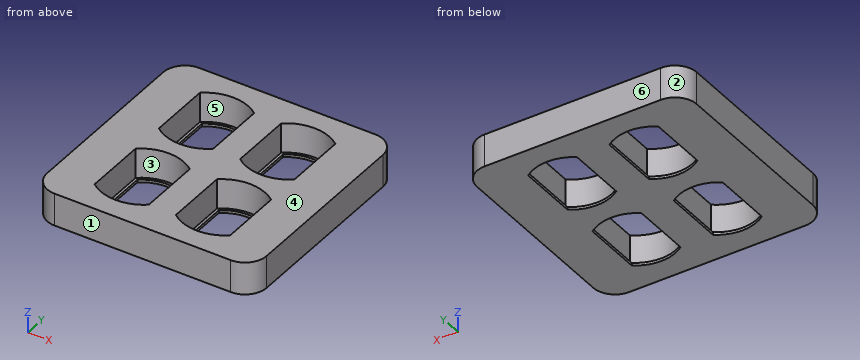
```python
from build123d import *

# Parameters (mm, degrees)
SKETCH1_W            = 81
SKETCH1_H            = 81
BOSS_EXTRUDE1_DEPTH  = 12
CUT_EXTRUDE1_DEPTH   = 11
CUT_EXTRUDE2_DEPTH   = 59.322379924
MIRROR3_COPY_1_DEPTH = 11
MIRROR3_COPY_2_DEPTH = 59.322379924
FILLET1_R            = 8


with BuildPart() as part:
    # Sketch1 → Boss-Extrude1 (new body)
    with BuildSketch(Plane.XY):
        Rectangle(SKETCH1_W, SKETCH1_H)
    extrude(amount=BOSS_EXTRUDE1_DEPTH)

    # Sketch2 → Cut-Extrude1 (cut)
    with BuildSketch(Plane.XY.offset(12)):
        with BuildLine():
            Line((-25, 6.5), (-25, 29.5))
            ThreePointArc((-25, 29.5), (-15, 33), (-5, 29.5))
            Line((-5, 29.5), (-5, 6.5))
            ThreePointArc((-5, 6.5), (-15, 3), (-25, 6.5))
        make_face()
    cut_extrude1 = extrude(amount=-CUT_EXTRUDE1_DEPTH, mode=Mode.SUBTRACT)

    # Sketch4 → Cut-Extrude2 (cut, through all)
    with BuildSketch(Plane.XY.offset(1)):
        with BuildLine():
            Line((-6, 6.991101213), (-6, 29.008898787))
            ThreePointArc((-6, 29.008898787), (-15, 32), (-24, 29.008898787))
            Line((-24, 29.008898787), (-24, 6.991101213))
            ThreePointArc((-24, 6.991101213), (-15, 4), (-6, 6.991101213))
        make_face()
    cut_extrude2 = extrude(amount=-CUT_EXTRUDE2_DEPTH, mode=Mode.SUBTRACT)

    # Mirror2: Cut-Extrude1, Cut-Extrude2 across plane
    add(cut_extrude1.mirror(Plane.ZX), mode=Mode.SUBTRACT)
    add(cut_extrude2.mirror(Plane.ZX), mode=Mode.SUBTRACT)

    # Mirror3: Cut-Extrude1, Cut-Extrude2 across plane
    add(cut_extrude1.mirror(Plane(origin=(0, 0, 0), x_dir=(0, 0, 1), z_dir=(1, 0, 0))), mode=Mode.SUBTRACT)
    add(cut_extrude2.mirror(Plane(origin=(0, 0, 0), x_dir=(0, 0, 1), z_dir=(1, 0, 0))), mode=Mode.SUBTRACT)

    # Mirror3 copy 1 sketch → Mirror3 copy 1 (cut)
    with BuildSketch(Plane(origin=(0, 0, 12), x_dir=(-1, 0, 0), z_dir=(0, 0, 1))):
        with BuildLine():
            Line((-25, 6.5), (-25, 29.5))
            ThreePointArc((-25, 29.5), (-15, 33), (-5, 29.5))
            Line((-5, 29.5), (-5, 6.5))
            ThreePointArc((-5, 6.5), (-15, 3), (-25, 6.5))
        make_face()
    extrude(amount=-MIRROR3_COPY_1_DEPTH, mode=Mode.SUBTRACT)

    # Mirror3 copy 2 sketch → Mirror3 copy 2 (cut, through all)
    with BuildSketch(Plane(origin=(0, 0, 1), x_dir=(-1, 0, 0), z_dir=(0, 0, 1))):
        with BuildLine():
            Line((-6, 6.991101213), (-6, 29.008898787))
            ThreePointArc((-6, 29.008898787), (-15, 32), (-24, 29.008898787))
            Line((-24, 29.008898787), (-24, 6.991101213))
            ThreePointArc((-24, 6.991101213), (-15, 4), (-6, 6.991101213))
        make_face()
    extrude(amount=-MIRROR3_COPY_2_DEPTH, mode=Mode.SUBTRACT)

    # Fillet1
    fillet1_edges = [part.edges().sort_by_distance(p)[0] for p in [
        (40.5, -40.5, 6),
        (-40.5, -40.5, 6),
        (-40.5, 40.5, 6),
        (40.5, 40.5, 6),
    ]]
    fillet(fillet1_edges, radius=FILLET1_R)


solid = part.part
```
Model file for the job. Use its own axes, mm. Face numbers are marked on the shaded views. A direction names the side the tool comes from. Give positions to 0.01 mm unless a question says otherwise; leave off trailing zeros. Write each loop counter-clockwise with the first axis right and the second up, starting at its lowest first coordinate (ties: lowest second). Pieces come first, ordered by that corner, then holes. Notation, with made-up numbers: M 30,4.25 L 69,4.25 A25 cw 69,40.25 Z; hole C -20,63 d11. An arc over 180 degrees is marked long. Use a Markdown table: item, result.
1) Tool access for the marked faces 5 and 6: list every direction of +Z, -Z, +X, -X, +Y, -Y with a clear straight run to the whole face (end or side of a thin tool).
Responses:
| item | result |
|---|---|
| face 5 | +Z |
| face 6 | +Z, -Z, +X, -X, +Y |
2) Cut at B-B (z = 5.5). List the corners of the cut face in (x, y), and give its area (3 significant figures).
Responses:
| item | result |
|---|---|
| outline | M -40.5,-32.5 A8 ccw -32.5,-40.5 L 32.5,-40.5 A8 ccw 40.5,-32.5 L 40.5,32.5 A8 ccw 32.5,40.5 L -32.5,40.5 A8 ccw -40.5,32.5 Z; hole M -25,-29.5 A16.04 ccw -5,-29.5 L -5,-6.5 A16.04 ccw -25,-6.5 Z; hole M -25,6.5 A16.04 ccw -5,6.5 L -5,29.5 A16.04 ccw -25,29.5 Z; hole M 5,-29.5 A16.04 ccw 25,-29.5 L 25,-6.5 A16.04 ccw 5,-6.5 Z; hole M 5,6.5 A16.04 ccw 25,6.5 L 25,29.5 A16.04 ccw 5,29.5 Z |
| area | 4,280 mm2 |
3) Pull direction Y, two halves, no side cores. Call the marked faces 1, 2, 3 and 4: +Y half, -Y half, draft (parallel to the pull), parting line (faces both ways), or undercut.
Responses:
| item | result |
|---|---|
| face 1 | -Y half |
| face 2 | +Y half |
| face 3 | undercut |
| face 4 | draft |
4) Pin check, flat tip, straight feed: pin 1 (16 mm diameter, centred on x = 18.5, y = -15.5, fed in from +Z). Stop position of the tip, or through.
Responses:
| item | result |
|---|---|
| pin 1 | stops at z = 12 |
5) Cut at C-C (x = -23). List the corners of the cut face in (y, z), and give its area (3 significant figures).
Responses:
| item | result |
|---|---|
| outline | M -40.5,0 L -29.7,0 L -29.7,1 L -30.86,1 L -30.86,12 L -40.5,12 Z; M -6.3,0 L 6.3,0 L 6.3,1 L 5.14,1 L 5.14,12 L -5.14,12 L -5.14,1 L -6.3,1 Z; M 29.7,0 L 40.5,0 L 40.5,12 L 30.86,12 L 30.86,1 L 29.7,1 Z |
| area | 359 mm2 |
6) Cut at A-A (y = -8). List the corners of the cut face in (x, z).
Responses:
| item | result |
|---|---|
| outline | M -40.5,0 L -24,0 L -24,1 L -25,1 L -25,12 L -40.5,12 Z; M -6,0 L 6,0 L 6,1 L 5,1 L 5,12 L -5,12 L -5,1 L -6,1 Z; M 24,0 L 40.5,0 L 40.5,12 L 25,12 L 25,1 L 24,1 Z |
7) Drill centre lines: line 1 (X direction, y = 23.5, z = 10.5); line 2 (Y direction, x = -7, z = 2.5); line 3 (Y direction, x = 20.5, z = 3.5). Where is each one in solid material? Low to high. Write a range as from..to.
Responses:
| item | result |
|---|---|
| line 1 | x = -40.5..-25, -5..5, 25..40.5 |
| line 2 | y = -40.5..-30.86, -5.14..5.14, 30.86..40.5 |
| line 3 | y = -40.5..-32.03, -3.97..3.97, 32.03..40.5 |
